Build history of the part. All positions in model axes, mm. Round coordinates to 2 decimals unless told otherwise and drop trailing zeros. Order: outer loops, then holes, each group sorted by start corner. A loop starts at its lowest first (then second) coordinate and runs counter-clockwise, first axis right, second up. Notation, with made-up numbers: (75, 42) -> (127, 42) arc R12 ccw to (127, 61) -> close; hole circle Ø7 at (2.5, -31.75). An arc over 180 degrees is marked (long way). Use a Markdown table: item, result. Add a question column.
Item 1: Pin check, flat tips, straight feed: pin 1 (4 mm diameter, centred on x = -0.5, z = -38, fed in from +Y); pin 2 (8 mm diameter, centred on y = -6.5, z = -31.5, fed in from -X); pin 3 (4 mm diameter, centred on y = -17, z = -8.5, fed in from +X). Stop position of each tip, or through.
Item 2: Slice it at C-C, the plane x = -11.5. Give the cut face in (y, z).
Item 3: Slice it at B-B, the plane z = -13. Give the cut face in (x, y).
Item 4: Slice it at A-A, the plane y = -5.5. Give the cut face in (x, z) (3 decimals), plus the area to 3 significant figures.
Item 5: Probe L1, parallel to Z at x = 50, y = -18.75; L2, parallel to Z at x = 55, y = -5.25; L3, parallel to X at y = -15, z = -16. List the from-to ranges inside material, lowest first.
from build123d import *

# Parameters (mm, degrees)
F0_W     = 20
F0_H     = 45
F1_DEPTH = 25


with BuildPart() as f1:
    # F0 (on Front) → F1 (new body)
    with BuildSketch(Plane.XZ):
        with BuildLine():
            Line((0, -45), (0, 0))
            ThreePointArc((0, 0), (-4.414268, -19.949802), (-16.832935, -36.175002))
            ThreePointArc((-16.832935, -36.175002), (-18.309855, -41.713915), (-13.612782, -45))
            Line((-13.612782, -45), (0, -45))
        make_face()
        with Locations((10, -22.5)):
            Rectangle(F0_W, F0_H)
        with BuildLine():
            ThreePointArc((65.491798, -35.414037), (38.466638, -23.204028), (20, 0))
            Line((20, 0), (20, -45))
            Line((20, -45), (63.499577, -45))
            ThreePointArc((63.499577, -45), (68.394974, -41.017395), (65.491798, -35.414037))
        make_face()
    extrude(amount=F1_DEPTH)


solid = f1.part
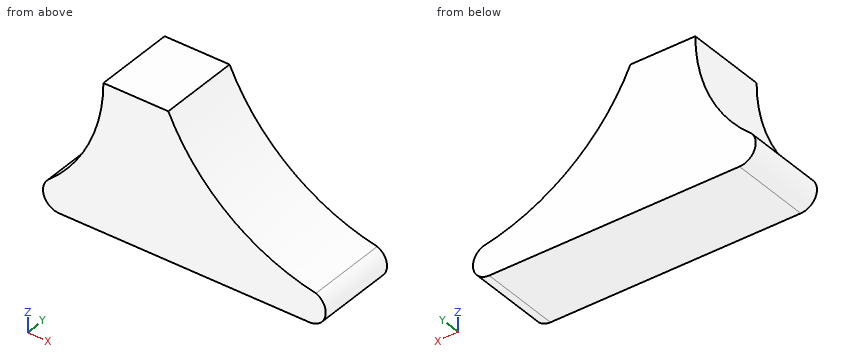
Check sheet entries:
| question | item | result |
|---|---|---|
| 1 | pin 1 | y = 0 |
| 1 | pin 2 | x = -16.05 |
| 1 | pin 3 | x = 26.18 |
| 2 | outline | (-25, -45) -> (0, -45) -> (0, -30.91) -> (-25, -30.91) -> close |
| 3 | outline | (-1.82, -25) -> (28.09, -25) -> (28.09, 0) -> (-1.82, 0) -> close |
| 4 | outline | (-16.833, -36.175) arc R5 ccw to (-13.613, -45) -> (63.5, -45) arc R5 ccw to (65.492, -35.414) arc R63.121 cw to (20, 0) -> (0, 0) arc R47.288 cw to start |
| 4 | area | 2,230 mm2 |
| 5 | L1 | -45 to -30.34 |
| 5 | L2 | -45 to -32.47 |
| 5 | L3 | -2.79 to 30.67 |
